Can you work these out from the model? Positions are in its coordinate system, mm. Face numbers are marked on the shaded views. A direction names the side the tool comes from. Round coordinates to 2 decimals unless told otherwise and drop trailing zeros. Order: outer loops, then holes, each group sorted by start corner. A loop starts at its lowest first (then second) coordinate and runs counter-clockwise, first axis right, second up. Notation, with made-up numbers: (-6, 30.25) - (49, 30.25) arc R33 cw to (49, 62.25) - close; hole circle Ø7 at (74, -30). An arc over 180 degrees is marked (long way). Write item = value, one per line.
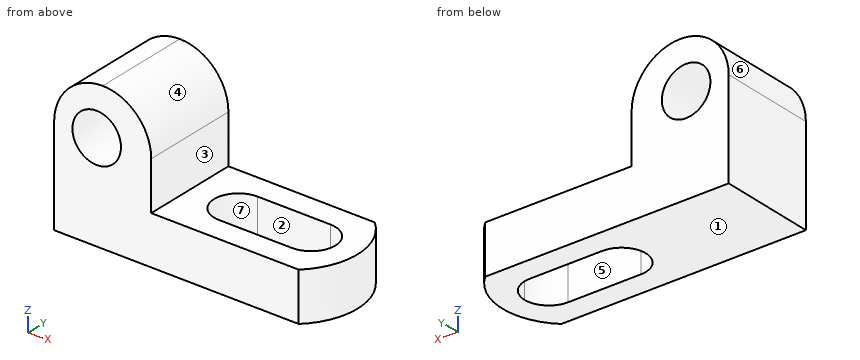
from build123d import *

# Parameters (mm, degrees)
F0_W      = 69.85
F0_H      = 38.1
F1_DEPTH  = 25.4
F2_W      = 44.45
F2_H      = 25.4
F3_DEPTH  = 25.4
F4_R      = 12.69999
F5_R      = 6.35
F6_DEPTH  = 25.4
F8_DEPTH  = 50.8
F10_DEPTH = 50.8


# Not quite as in the source:
# - a fillet or chamfer is up to 0.001 mm smaller than in the source, because OpenCascade refuses the exact size


with BuildPart() as f1:
    # F0 (on Front) → F1 (new body)
    with BuildSketch(Plane.XZ):
        with Locations((34.925, 19.05)):
            Rectangle(F0_W, F0_H)
    extrude(amount=F1_DEPTH)

    # F2 (on face) → F3 (cut)
    with BuildSketch(Plane.XZ.offset(25.4)):
        with Locations((47.625, 25.4)):
            Rectangle(F2_W, F2_H)
    extrude(amount=-F3_DEPTH, mode=Mode.SUBTRACT)

    # F4 (radius 12.7 in the source; OpenCascade refuses exactly that, so slightly less here)
    f4_edges = [f1.edges().sort_by_distance(p)[0] for p in [
        (25.4, -12.7, 38.1),
        (0, -12.7, 38.1),
    ]]
    fillet(f4_edges, radius=F4_R)

    # F5 (on face) → F6 (cut)
    with BuildSketch(Plane.XZ.offset(25.4)):
        with Locations((11.1332936212, 25.4)):
            Circle(F5_R)
    extrude(amount=-F6_DEPTH, mode=Mode.SUBTRACT)

    # F7 (on face) → F8 (cut)
    with BuildSketch(Plane.XY.offset(12.7)):
        with BuildLine():
            ThreePointArc((38.1, -19.05), (42.5901280605, -17.1901280605), (44.45, -12.7))
            ThreePointArc((44.45, -12.7), (42.5901280605, -8.2098719395), (38.1, -6.35))
            ThreePointArc((38.1, -6.35), (31.75, -12.7), (38.1, -19.05))
        make_face()
        with BuildLine():
            ThreePointArc((38.1, -6.35), (42.5901280605, -8.2098719395), (44.45, -12.7))
            ThreePointArc((44.45, -12.7), (42.5901280605, -17.1901280605), (38.1, -19.05))
            Line((38.1, -19.05), (57.15, -19.05))
            ThreePointArc((57.15, -19.05), (50.8, -12.7), (57.15, -6.35))
            Line((57.15, -6.35), (38.1, -6.35))
        make_face()
        with BuildLine():
            ThreePointArc((63.5, -12.7), (61.6401280605, -8.2098719395), (57.15, -6.35))
            ThreePointArc((57.15, -6.35), (50.8, -12.7), (57.15, -19.05))
            ThreePointArc((57.15, -19.05), (61.6401280605, -17.1901280605), (63.5, -12.7))
        make_face()
    extrude(amount=-F8_DEPTH, mode=Mode.SUBTRACT)

    # F9 (on face) → F10 (cut)
    with BuildSketch(Plane.XY.offset(12.7)):
        with BuildLine():
            ThreePointArc((63.6959075928, 0), (69.3784721841, -12.6381087117), (63.9796331525, -25.4))
            Line((63.9796331525, -25.4), (69.85, -25.4))
            Line((69.85, -25.4), (69.85, 0))
            Line((69.85, 0), (63.6959075928, 0))
        make_face()
    extrude(amount=-F10_DEPTH, mode=Mode.SUBTRACT)


solid = f1.part
(1) If we section it at B-B (y = -14.25): State how many separate pieces and enclosed holes the cut face has, plus the area to 3 significant figures.
Computed:
separate_pieces = 2
enclosed_holes = 1
area = 931 mm^2
(2) If we section it at A-A (x = 41.5): Write out the boundary of the cut face in (y, z), plus the area to 3 significant figures.
Computed:
outline = (-25.4, 0) - (-19.05, 0) - (-19.05, 12.7) - (-25.4, 12.7) - close; (-6.35, 0) - (0, 0) - (0, 12.7) - (-6.35, 12.7) - close
area = 161 mm^2
(3) If we section it at D-D (z = 11): Write out the boundary of the cut face in (x, y), plus the area to 3 significant figures.
Computed:
outline = (0, -25.4) - (63.98, -25.4) arc R17.33 ccw to (63.7, 0) - (0, 0) - close; hole (38.1, -19.05) - (57.15, -19.05) arc R6.35 ccw to (57.15, -6.35) - (38.1, -6.35) arc R6.35 ccw to start
area = 1,350 mm^2
(4) Thinking about a two-plate mould opening in X: for the marked faces 4, 5, 6 and 7, which applies, +X half, -X half, draft (parallel to the pull), parting line (faces both ways), or undercut?
Computed:
face_4 = +X half
face_5 = undercut
face_6 = -X half
face_7 = undercut
(5) If I drill on line 1 (Y direction, x = 45, z = 4); line 2 (Z direction, x = 40, y = -3.75); line 3 (X direction, y = -8, z = 15), over which ranges is the centre line in solid material (lowest first)? Write a range as from..to.
Computed:
line_1 = -25.4..-19.05, -6.35..0
line_2 = 0..12.7
line_3 = 0..25.4
(6) Will these pins go through, and if not, where does the flat tip stop? P1, Ø6, axis at x = 54.5, y = -13.5, coming from the -Z side; P2, Ø10, axis at x = 37.5, y = -3.5, coming from the +Z side; P3, Ø8, axis at y = -14.5, z = 31, coming from the +X side; P4, Ø4, axis at x = 19.5, y = -13, coming from the +Z side.
Computed:
P1 = through
P2 = 12.7
P3 = 25.3
P4 = 37.16
(7) If we section it at C-C (z = 29): Write out the boundary of the cut face in (x, y).
Computed:
outline = (0.52, -25.4) - (5.9, -25.4) - (5.9, 0) - (0.52, 0) - close; (16.36, -25.4) - (24.88, -25.4) - (24.88, 0) - (16.36, 0) - close
(8) On a 3-axis mill with a long thin cutter (end or side, diameter ignored), from which of +Z, -Z, +X, -X, +Y, -Y can I reach the whole of each face in a straight line? I mean the marked faces 1, 2 and 3. Say none if no direction works.
Computed:
face_1 = -Z, +X, -X, +Y, -Y
face_2 = +Z, -Z
face_3 = +Z, +X, +Y, -Y
